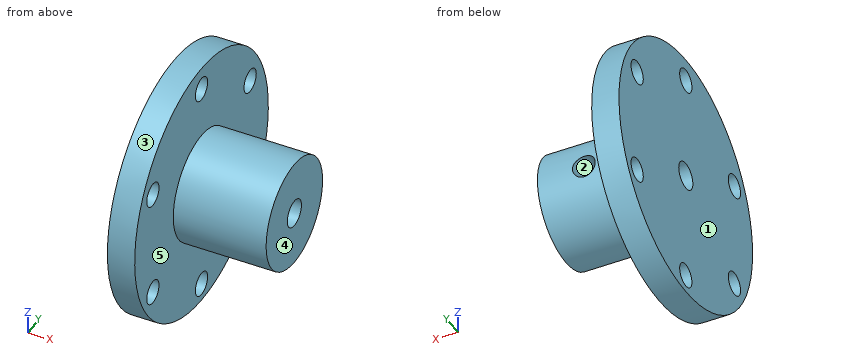
from build123d import *

# Parameters (mm, degrees)
ESQUISSE2_R             = 2.6
ENL_V_MAT_EXTRU_1_DEPTH = 10
ESQUISSE3_R             = 2.5
ENL_V_MAT_EXTRU_2_DEPTH = 10


with BuildPart() as part:
    # Esquisse1 → Révolution1 (revolve)
    with BuildSketch(Plane.XY, mode=Mode.PRIVATE) as r_volution1_sk:
        Polygon((-39.661027285, 12), (-60.061027285, 12), (-60.061027285, 28.4), (-66.061027285, 28.4), (-66.061027285, 3), (-39.661027285, 3), align=None)
    revolve(r_volution1_sk.sketch.rotate(Axis((54.367533201, 0, 0), (-1, 0, 0)), 90), axis=Axis((54.367533201, 0, 0), (-1, 0, 0)))

    # Esquisse2 → Enlèv. mat.-Extru.1 (cut)
    with BuildSketch(Plane(origin=(-60.061027285, 0, 0), x_dir=(0, 0, -1), z_dir=(1, 0, 0))):
        with Locations((-23.344444301, 0)):
            Circle(ESQUISSE2_R)
        with Locations((-11.406944301, 20.676356515)):
            Circle(ESQUISSE2_R)
        with Locations((12.468055699, 20.676356515)):
            Circle(ESQUISSE2_R)
        with Locations((24.405555699, 0)):
            Circle(ESQUISSE2_R)
        with Locations((12.468055699, -20.676356515)):
            Circle(ESQUISSE2_R)
        with Locations((-11.406944301, -20.676356515)):
            Circle(ESQUISSE2_R)
    extrude(amount=-ENL_V_MAT_EXTRU_1_DEPTH, mode=Mode.SUBTRACT)

    # Esquisse3 → Enlèv. mat.-Extru.2 (cut)
    with BuildSketch(Plane(origin=(0, 12, 0), x_dir=(-1, 0, 0), z_dir=(0, -1, 0))):
        with Locations((49.861027285, 0)):
            Circle(ESQUISSE3_R)
    extrude(amount=ENL_V_MAT_EXTRU_2_DEPTH, mode=Mode.SUBTRACT)


solid = part.part
Here's how the part is built. I have some questions about the finished solid (model axes, mm). Face numbers are marked on the shaded views. A direction names the side the tool comes from. Give positions to 0.01 mm unless a question says otherwise; leave off trailing zeros. Loops run counter-clockwise (first coordinate to the right, second up) from the corner with the lowest first, then second, coordinate; pieces in that order, holes last. Notation, with made-up numbers: (-18, 17) -> (7, 17) arc R37 ccw to (7, 54) -> close; hole circle Ø10 at (-9.5, -3.5). An arc over 180 degrees is marked (long way). Answer as a JSON object with one key per item and string values. Group by question number.
Item 1: Imagine slicing it at A-A on z = 0. Write out the boundary of the cut face in (x, y), then the cut area to 3 significant figures.
Item 2: Imagine slicing it at D-D on y = 21.5. Write out the boundary of the cut face in (x, z).
Item 3: Will these pins go through, and if not, where does the flat tip stop? pin 1 (10 mm diameter, centred on x = -42.5, z = 15, fed in from -Y); pin 2 (4.5 mm diameter, centred on y = 0, z = -24.41, fed in from +X); pin 3 (4 mm diameter, centred on x = -49.86, z = 0, fed in from +Y); pin 4 (12 mm diameter, centred on x = -54, z = 7.5, fed in from -Y).
Item 4: On a 3-axis mill with a long thin cutter (end or side, diameter ignored), from which of +Z, -Z, +X, -X, +Y, -Y can I reach the whole of each face in a straight line? I mean the marked faces 4 and 5. Say none if no direction works.
Item 5: Imagine slicing it at C-C on z = -24.5. Write out the boundary of the cut face in (x, y), then the cut area to 3 significant figures.
Item 6: Thinking about a two-plate mould opening in Z: for the marked faces 1, 2 and 3, which applies, pulls with the +Z half, pulls with the -Z half, needs draft (parallel to the pull), parting line crosses it, or undercut?
Item 7: I need wall thicknesses on L1, parallel to X at y = 16, z = 19.5; L2, parallel to Y at x = -43.5, z = 2.5; L3, parallel to Y at x = -62.5, z = -0.5. Which ranges of each line are inside material? Lowest first, please.
Item 8: Imagine slicing it at B-B on y = 0. Write out the boundary of the cut face in (x, z), then the cut area to 3 significant figures.
Answer list:
{
 "1": {"outline": "(-66.06, -28.4) -> (-60.06, -28.4) -> (-60.06, -12) -> (-39.66, -12) -> (-39.66, -3) -> (-66.06, -3) -> close; (-66.06, 3) -> (-52.36, 3) -> (-52.36, 12) -> (-60.06, 12) -> (-60.06, 28.4) -> (-66.06, 28.4) -> close; (-47.36, 3) -> (-39.66, 3) -> (-39.66, 12) -> (-47.36, 12) -> close", "area": "627 mm2"},
 "2": {"outline": "(-66.06, -18.56) -> (-60.06, -18.56) -> (-60.06, -14.93) -> (-66.06, -14.93) -> close; (-66.06, -10) -> (-60.06, -10) -> (-60.06, 8.94) -> (-66.06, 8.94) -> close; (-66.06, 13.87) -> (-60.06, 13.87) -> (-60.06, 18.56) -> (-66.06, 18.56) -> close"},
 "3": {"pin 1": "stops at y = -6.63", "pin 2": "passes through", "pin 3": "stops at y = -2.24", "pin 4": "stops at y = -11.91"},
 "4": {"face 4": "+Z, -Z, +X, +Y, -Y", "face 5": "+X"},
 "5": {"outline": "(-66.06, -14.36) -> (-60.06, -14.36) -> (-60.06, -2.6) -> (-66.06, -2.6) -> close; (-66.06, 2.6) -> (-60.06, 2.6) -> (-60.06, 14.36) -> (-66.06, 14.36) -> close", "area": "141 mm2"},
 "6": {"face 1": "needs draft", "face 2": "undercut", "face 3": "parting line crosses it"},
 "7": {"L1": "x = -66.06 to -60.06", "L2": "y = -11.74 to -1.66, 1.66 to 11.74", "L3": "y = -28.4 to -2.96, 2.96 to 28.4"},
 "8": {"outline": "(-66.06, -28.4) -> (-60.06, -28.4) -> (-60.06, -27.01) -> (-66.06, -27.01) -> close; (-66.06, -21.81) -> (-60.06, -21.81) -> (-60.06, -12) -> (-39.66, -12) -> (-39.66, -3) -> (-66.06, -3) -> close; (-66.06, 3) -> (-39.66, 3) -> (-39.66, 12) -> (-60.06, 12) -> (-60.06, 20.74) -> (-66.06, 20.74) -> close; (-66.06, 25.94) -> (-60.06, 25.94) -> (-60.06, 28.4) -> (-66.06, 28.4) -> close", "area": "610 mm2"}
}
